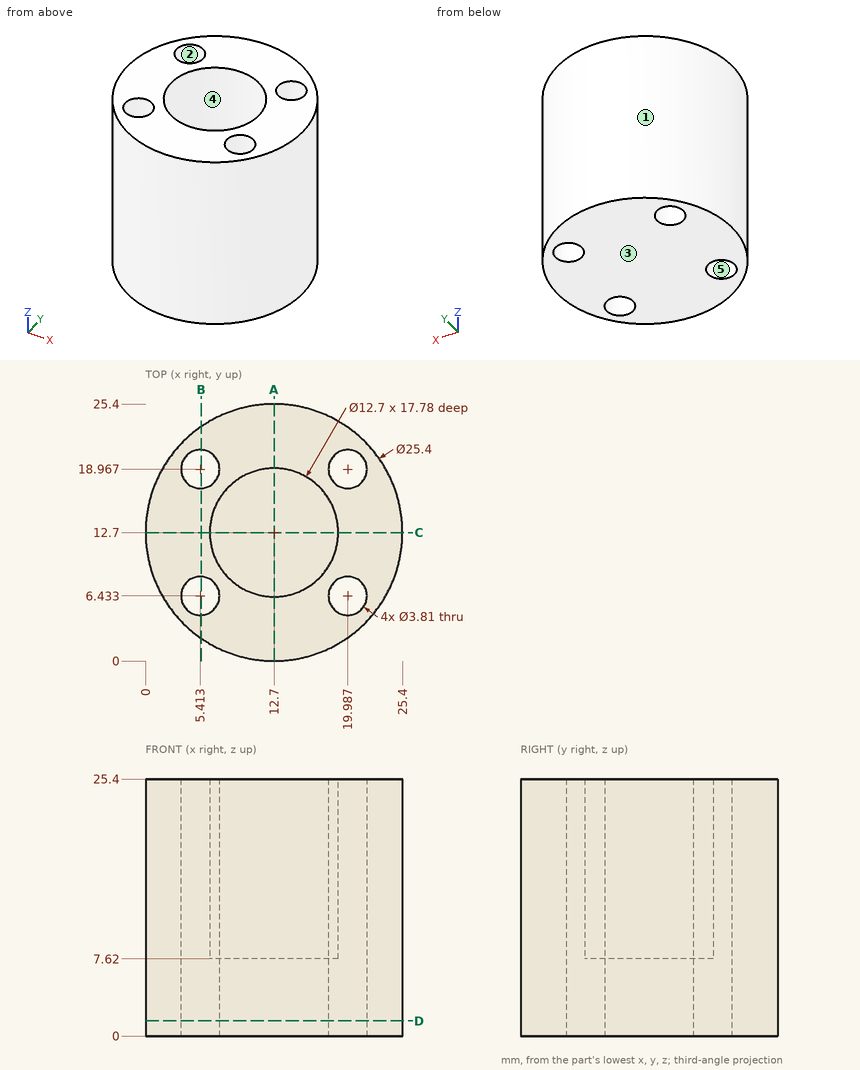
Check sheet for the drawn part. Datum: minimum x, y, z corner. Units: mm. A direction names the side the tool comes from. Coordinates: 2 decimals unless noted, no trailing zeros. Write each loop counter-clockwise with the first axis right and the second up, starting at its lowest first coordinate (ties: lowest second). Pieces come first, ordered by that corner, then holes. Notation, with made-up numbers: M -30,-17 L -15,-17 A21 cw -15,14 Z; hole C 82,40.25 d11. An arc over 180 degrees is marked long. One line per item, written item: value.
Item 1: Gauge pin test, flat ends, axial feed: pin 1 Ø1 at (y, z) = (23, 14) entering from -X; pin 2 Ø3 at (x, z) = (17, 15) entering from +Y; pin 3 Ø6.5 at (x, y) = (11.5, 11) entering from +Z; pin 4 Ø3 at (x, y) = (5.41, 6.43) entering from +Z. Record the tip position at first contact, or that the pin passes through.
Check sheet entries:
pin 1: stops at x = 4.62
pin 2: stops at y = 25.09
pin 3: stops at z = 7.62
pin 4: passes through
Item 2: Mould release check, pull along X, two halves, no side actions. Record for the marked faces 1, 2 and 3: pulls with the +X half, pulls with the -X half, needs draft (parallel to the pull), parting line crosses it, or undercut.
Check sheet entries:
face 1: parting line crosses it
face 2: undercut
face 3: needs draft
Item 3: Scan lines: line 1 along X through (y, z) = (17.25, 15.5) (1 decimal); line 2 along Y through (x, z) = (3.75, 4.5) (1 decimal); line 3 along X through (y, z) = (6.25, 4.75). Record each from-to range of solid material in increasing order.
Check sheet entries:
line 1: x = 0.8 to 4.6, 6.2 to 8.3, 17.1 to 19.2, 20.8 to 24.6
line 2: y = 3.7 to 5.5, 7.4 to 18, 19.9 to 21.7
line 3: x = 1.76 to 3.52, 7.31 to 18.09, 21.88 to 23.64
Item 4: Section check D-D, the plane z = 1.5. Record the boundary of the cut face in (x, y) (1 decimal).
Check sheet entries:
outline: C 12.7,12.7 d25.4; hole C 5.4,6.4 d3.8; hole C 5.4,19 d3.8; hole C 20,6.4 d3.8; hole C 20,19 d3.8
Item 5: Access from +Z, -Z, +X, -X, +Y, -Y to the whole of each face (thin tool, end or side, straight path). Record for the marked faces 4 and 5.
Check sheet entries:
face 4: +Z
face 5: +Z, -Z
Item 6: Section check A-A, the plane x = 12.7. Record the boundary of the cut face in (y, z), plus the area to 3 significant figures.
Check sheet entries:
outline: M 0,0 L 25.4,0 L 25.4,25.4 L 19.05,25.4 L 19.05,7.62 L 6.35,7.62 L 6.35,25.4 L 0,25.4 Z
area: 419 mm^2
Item 7: Section check B-B, the plane x = 5.5. Record the boundary of the cut face in (y, z), plus the area to 3 significant figures.
Check sheet entries:
outline: M 2.24,0 L 4.53,0 L 4.53,25.4 L 2.24,25.4 Z; M 8.34,0 L 17.06,0 L 17.06,25.4 L 8.34,25.4 Z; M 20.87,0 L 23.16,0 L 23.16,25.4 L 20.87,25.4 Z
area: 338 mm^2
